Part model, mm, in its own coordinate system. Give positions to 0.01 mm unless a question says otherwise; leave off trailing zeros. Write each loop counter-clockwise with the first axis right and the second up, starting at its lowest first coordinate (ties: lowest second). Pieces come first, ordered by that corner, then holes. Notation, with made-up numbers: (-20.75, -34.75) - (3.25, -34.75) arc R6 ccw to (3.25, -24.75) - close; hole circle Ø11 at (16.25, 35.5). An arc over 180 degrees is marked (long way). Answer as a JSON object with one key per item and string values. Group by question number.
Autodesk Fusion 360 part; units mm, degrees
sketch "Sketch1" plane through (0, 0, 0) normal (1, 0, 0) x (0, 0, -1)
  line L0 (0, 0) -> (-50, 0)
  line L1 (-50, 0) -> (-50, 10)
  line L2 (-50, 10) -> (0, 10)
  line L3 (0, 10) -> (0, 0)
  line L4 (0, 0) -> (65, 0)
  line L5 (65, 0) -> (65, 10)
  line L6 (65, 10) -> (0, 10)
  line L7 (0, 10) -> (0, 0)
  line L8 (-50, 0) -> (-115, 0)
  line L9 (-115, 0) -> (-115, 10)
  line L10 (-115, 10) -> (-50, 10)
  line L11 (-50, 10) -> (-50, 0)
  dimension "d1" = 50
  dimension "d2" = 10
  dimension "d3" = 65
  dimension "d4" = 65
  dimension "d5" = 10
  dimension "d6" = 10
extrude "Extrude1" add sketch "Sketch1" along normal blind 130
extrude "Extrude2" add sketch "Sketch1" against normal blind 10 contours L0 L1 L2 L3 L7 L11
sketch "Sketch2" plane through (130, 0, 0) normal (1, 0, 0) x (0, 0, -1)
  line L0 (-115, 0) -> (65, 0)
  line L1 (65, 0) -> (65, 10)
  line L2 (65, 10) -> (-115, 10)
  line L3 (-115, 10) -> (-115, 0)
  line L4 (-50, 0) -> (0, 0)
  line L5 (0, 0) -> (0, 10)
  line L6 (0, 10) -> (-50, 10)
  line L7 (-50, 10) -> (-50, 0)
extrude "Extrude3" add sketch "Sketch2" along normal blind 10 contours L0 L2 L4 L5 L6 L7
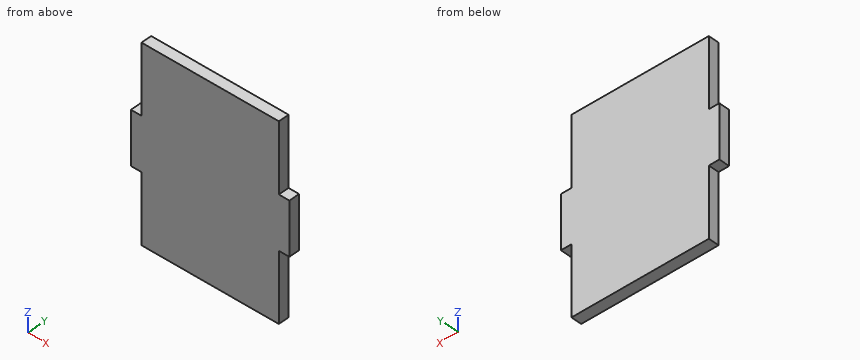
1) Drop flat-ended pins along their axis: P1, Ø3, axis at x = -3, y = 5.5, coming from the +Z side; P2, Ø5, axis at y = 3, z = -43.5, coming from the -X side; P3, Ø4, axis at y = 7, z = -43.5, coming from the +X side; P4, Ø12, axis at x = 21, z = 73, coming from the -Y side. Give the stop position or say it passes through.
2) Drill centre line: line 1 along X through (y, z) = (8, -19). Where is it in solid material? Low to high. Write a range as from..to.
3) Saw through at A-A (y = 6.5). List the corners of the cut face in (x, z), and give its area (3 significant figures).
4) Saw through at B-B (z = 75.5). List the corners of the cut face in (x, y), and give its area (3 significant figures).
Checks:
{
 "1": {"P1": "z = 50", "P2": "x = 0", "P3": "x = 130", "P4": "y = 0"},
 "2": {"line 1": "0..130"},
 "3": {"outline": "(-10, 0) - (0, 0) - (0, -65) - (130, -65) - (130, 0) - (140, 0) - (140, 50) - (130, 50) - (130, 115) - (0, 115) - (0, 50) - (-10, 50) - close", "area": "24,400 mm2"},
 "4": {"outline": "(0, 0) - (130, 0) - (130, 10) - (0, 10) - close", "area": "1,300 mm2"}
}
